The listing builds one solid part. Answer for the finished solid, in the listing's coordinates (mm). A direction names the side the tool comes from. Coordinates: 2 decimals unless noted, no trailing zeros. Order: outer loops, then holes, each group sorted by start corner. A loop starts at its lowest first (then second) coordinate and runs counter-clockwise, first axis right, second up. Notation, with made-up numbers: (56, 54.5) -> (93, 54.5) arc R28 ccw to (93, 78.5) -> close; hole circle Ø11 at (89.5, -5). An arc over 180 degrees is marked (long way). Answer in a Markdown table with one row per item.
Autodesk Inventor part; units mm, degrees
ref_plane "YZ Plane" through (0, 0, 0) normal (1, 0, 0) x (0, 1, 0)
ref_plane "XZ Plane" through (0, 0, 0) normal (0, 1, 0) x (-1, 0, 0)
ref_plane "XY Plane" through (0, 0, 0) normal (0, 0, 1) x (1, 0, 0)
sketch "Sketch1" plane through (0, 0, 0) normal (0, 0, 1) x (1, 0, 0)
  arc A0 (63.3108, 19.3076) -> (65.1069, 15.7154) centre (69.597, 20.2056) ccw
  arc A1 (63.3108, 19.3076) -> (56.1947, 27.2004) centre (53.8815, 17.9605) ccw
  arc A2 (56.1947, 27.2004) -> (54.6834, 21.1637) centre (55.439, 24.182) ccw
  arc A3 (50.6775, 17.1623) -> (54.6834, 21.1637) centre (53.8815, 17.9605) ccw
  arc A4 (50.6775, 17.1623) -> (44.9626, 17.9641) centre (47.6583, 16.4101) ccw
  arc A5 (39.4613, 14.7855) -> (44.9626, 17.9641) centre (39.4613, 21.1355) ccw
  line L0 (32.3778, 14.7855) -> (39.4613, 14.7855)
  arc A6 (26.8779, 17.9617) -> (32.3778, 14.7855) centre (32.3778, 21.1355) ccw
  arc A7 (26.8779, 17.9617) -> (21.1641, 17.1604) centre (24.1829, 16.4065) ccw
  arc A8 (17.1604, 21.1641) -> (21.1641, 17.1604) centre (17.9605, 17.9605) ccw
  arc A9 (17.1604, 21.1641) -> (15.6526, 27.2017) centre (16.4065, 24.1829) ccw
  arc A10 (15.6526, 27.2017) -> (8.5312, 19.3076) centre (17.9605, 17.9605) ccw
  arc A11 (6.7352, 15.7154) -> (8.5312, 19.3076) centre (2.2451, 20.2056) ccw
  line L1 (2.2451, 11.2253) -> (6.7352, 15.7154)
  arc A12 (-1.347, 9.4293) -> (2.2451, 11.2253) centre (-2.2451, 15.7154) ccw
  arc A13 (-1.347, 9.4293) -> (-9.2412, 2.3079) centre (0, 0) ccw
  arc A14 (-9.2412, 2.3079) -> (-3.2036, 0.8001) centre (-6.2224, 1.554) ccw
  arc A15 (0.8001, -3.2036) -> (-3.2036, 0.8001) centre (0, 0) ccw
  arc A16 (0.8001, -3.2036) -> (2.3079, -9.2412) centre (1.554, -6.2224) ccw
  arc A17 (2.3079, -9.2412) -> (4.0839, -8.6051) centre (0, 0) ccw
  arc A18 (15.7006, -6.4053) -> (4.0839, -8.6051) centre (14.0949, -29.6986) ccw
  arc A19 (15.7006, -6.4053) -> (18.5812, -1.6996) centre (15.9135, -3.3011) ccw
  arc A20 (24.2432, -1.6996) -> (18.5812, -1.6996) centre (21.4122, 0) ccw
  arc A21 (24.2432, -1.6996) -> (29.5786, -4.9026) centre (26.9109, -3.3011) ccw
  arc A22 (29.5786, -4.9026) -> (30.5871, -2.5587) centre (21.4122, 0) ccw
  arc A23 (36.7037, 2.0855) -> (30.5871, -2.5587) centre (36.7037, -4.2645) ccw
  line L2 (56.5506, 2.0855) -> (36.7037, 2.0855)
  arc A24 (62.6672, -2.5587) -> (56.5506, 2.0855) centre (56.5506, -4.2645) ccw
  arc A25 (62.6672, -2.5587) -> (69.5342, -9.2412) centre (71.842, 0) ccw
  arc A26 (69.5342, -9.2412) -> (71.042, -3.2036) centre (70.2881, -6.2224) ccw
  arc A27 (75.0457, 0.8001) -> (71.042, -3.2036) centre (71.842, 0) ccw
  arc A28 (75.0457, 0.8001) -> (81.0832, 2.3079) centre (78.0644, 1.554) ccw
  arc A29 (81.0832, 2.3079) -> (73.1891, 9.4293) centre (71.842, 0) ccw
  arc A30 (69.597, 11.2253) -> (73.1891, 9.4293) centre (74.0871, 15.7154) ccw
  line L3 (65.1069, 15.7154) -> (69.597, 11.2253)
extrude "Extrusion1" add sketch "Sketch1" against normal blind 25.273
properties part number "am-0212" material "Aluminum-6061"
(1) A cutting plane is placed at B-B, the plane x = 58. Determine the outline of the cut face in (y, z).
Check values:
| item | result |
|---|---|
| outline | (1.92, -25.27) -> (26.55, -25.27) -> (26.55, 0) -> (1.92, 0) -> close |
(2) Flat-ended cylindrical pins translate along their axes: pin 1 (5.5 mm diameter, centred on x = 0, y = 0, fed in from -Z); pin 2 (4 mm diameter, centred on x = 34.5, z = -12, fed in from +Y); pin 3 (10 mm diameter, centred on x = 44, z = -14, fed in from -Y); pin 4 (5 mm diameter, centred on x = 4.5, y = 10.5, fed in from +Z). Find the tip coordinate at first contact, or state that the pin passes through.
Check values:
| item | result |
|---|---|
| pin 1 | through |
| pin 2 | y = 14.79 |
| pin 3 | y = 2.09 |
| pin 4 | z = 0 |
(3) Which of the six approach directions +Z, -Z, +X, -X, +Y, -Y give full straight-line access (tool end or side, diameter ignored) to faces 1 (the flat face through (35, 9, 0)), 2 (the cylindrical face through (42.598, 15.614, -12.46)), 3 (the cylindrical face through (30.155, -3.781, -12.46))?
Check values:
| item | result |
|---|---|
| face 1 | +Z, +X, -X, +Y, -Y |
| face 2 | +Z, -Z, +Y |
| face 3 | +Z, -Z, -Y |
(4) Find the intervals of material crossed by line 1 along X through (y, z) = (-5, -6.5); line 2 along X through (y, z) = (17.5, -12.75); line 3 along X through (y, z) = (-3, -5.25), in increasing order. Write a range as from..to.
Check values:
| item | result |
|---|---|
| line 1 | -1.31..18.52, 24.3..29.52, 63.73..73.15 |
| line 2 | 7.99..14.69, 21.27..27.17, 44.67..50.57, 57.15..63.85 |
| line 3 | 1.38..19.01, 23.81..30.45, 62.8..70.46 |
(5) A cutting plane is placed at A-A, the plane y = -0.5. Determine the outline of the cut face in (x, z).
Check values:
| item | result |
|---|---|
| outline | (-8.56, -25.27) -> (-3.89, -25.27) -> (-3.89, 0) -> (-8.56, 0) -> close; (3.26, -25.27) -> (18.15, -25.27) -> (18.15, 0) -> (3.26, 0) -> close; (24.68, -25.27) -> (31.59, -25.27) -> (31.59, 0) -> (24.68, 0) -> close; (61.66, -25.27) -> (68.58, -25.27) -> (68.58, 0) -> (61.66, 0) -> close; (75.73, -25.27) -> (80.4, -25.27) -> (80.4, 0) -> (75.73, 0) -> close |
